Input: part model. Units: mm. Frame: model coordinates. A direction names the side the tool comes from. Round coordinates to 2 decimals unless told otherwise and drop trailing zeros. Loops run counter-clockwise (first coordinate to the right, second up) from the corner with the lowest first, then second, coordinate; pieces in that order, holes last.
(1) First-contact query: pin 1 Ø22.5 at (y, z) = (56.5, -24.5) entering from -X; pin 2 Ø12 at (x, y) = (30.5, 42) entering from -Z; pin 3 Ø6 at (x, z) = (44.5, -2.5) entering from -Y. Flat tips, straight axial feed; report the tip coordinate or a pass-through.
(2) Access query for faces 1 (the face through (50, 49, -22)), 2 (the face through (39.9, 100, 0.3)). Directions: +Z, -Z, +X, -X, +Y, -Y. A direction counts if a zero-diameter tool reaches every point of the face in a straight line with its end or side. Return the directions, or none.
(3) Cut plane A-A, the plane y = 19. Output: boundary loops of the cut face in (x, z), and give its area (3 significant figures).
(4) Cut plane D-D, the plane x = 13.5. Output: boundary loops of the cut face in (y, z).
(5) Cut plane B-B, the plane x = 22. Output: boundary loops of the cut face in (y, z).
(6) Cut plane C-C, the plane z = -26. Output: boundary loops of the cut face in (x, y).
(7) Line query: line 1 (Z direction, x = 4.5, y = 69); line 2 (X direction, y = 53, z = -23.5). Output: solid intervals per line, ascending.
from build123d import *

# Parameters (mm, degrees)
BOSS_EXTRUDE2_DEPTH = 100
CUT_EXTRUDE1_DEPTH  = 100


with BuildPart() as part:
    # Sketch1 → Boss-Extrude2 (new body)
    with BuildSketch(Plane(origin=(0, 0, 0), x_dir=(1, 0, 0), z_dir=(0, 1, 0))):
        Polygon((0, 0), (50, 0), (50, 45), (55, 45), (55, -5), (0, -5), align=None)
    extrude(amount=BOSS_EXTRUDE2_DEPTH)

    # Sketch2 → Cut-Extrude1 (cut)
    with BuildSketch(Plane(origin=(0, 0, 0), x_dir=(-1, 0, 0), z_dir=(0, 0, -1))):
        with BuildLine():
            ThreePointArc((-25, 28), (-31, 22), (-25, 16))
            Line((-25, 16), (-25, 28))
        make_face()
        with BuildLine():
            Line((-25, 28), (-25, 16))
            ThreePointArc((-25, 16), (-20.757359313, 17.757359313), (-19, 22))
            ThreePointArc((-19, 22), (-20.757359313, 26.242640687), (-25, 28))
        make_face()
        with BuildLine():
            ThreePointArc((-25, 84), (-31, 78), (-25, 72))
            Line((-25, 72), (-25, 84))
        make_face()
        with BuildLine():
            Line((-25, 84), (-25, 72))
            ThreePointArc((-25, 72), (-20.757359313, 73.757359313), (-19, 78))
            ThreePointArc((-19, 78), (-20.757359313, 82.242640687), (-25, 84))
        make_face()
    extrude(amount=-CUT_EXTRUDE1_DEPTH, mode=Mode.SUBTRACT)


solid = part.part
Reported:
1. pin 1: stops at x = 50
1. pin 2: stops at z = 0
1. pin 3: stops at y = 0
2. face 1: -Z, -X, +Y, -Y
2. face 2: +Z, -Z, +X, -X, +Y
3. outline: (0, 0) - (19.8, 0) - (19.8, 5) - (0, 5) - close; (30.2, 0) - (50, 0) - (50, -45) - (55, -45) - (55, 5) - (30.2, 5) - close
3. area: 448 mm2
4. outline: (0, 0) - (100, 0) - (100, 5) - (0, 5) - close
5. outline: (0, 0) - (16.8, 0) - (16.8, 5) - (0, 5) - close; (27.2, 0) - (72.8, 0) - (72.8, 5) - (27.2, 5) - close; (83.2, 0) - (100, 0) - (100, 5) - (83.2, 5) - close
6. outline: (50, 0) - (55, 0) - (55, 100) - (50, 100) - close
7. line 1: z = 0 to 5
7. line 2: x = 50 to 55
